Here's how the part is built. I have some questions about the finished solid (model axes, mm). A direction names the side the tool comes from. Round coordinates to 2 decimals unless told otherwise and drop trailing zeros. Order: outer loops, then holes, each group sorted by start corner. A loop starts at its lowest first (then second) coordinate and runs counter-clockwise, first axis right, second up.
```python
from build123d import *

# Parameters (mm, degrees)
BOSS_EXTRU_1_DEPTH      = 12
BOSS_EXTRU_1_DEPTH_BACK = 6
ENL_V_MAT_EXTRU_1_DEPTH = 168.845911478
BOSS_EXTRU_2_DEPTH      = 20
ENL_V_MAT_EXTRU_2_DEPTH = 169.042623851
ESQUISSE5_R             = 1.9
ENL_V_MAT_EXTRU_3_DEPTH = 10
CONG_1_R                = 3
CONG_2_R                = 1.5


with BuildPart() as part:
    # Esquisse1 → Boss.-Extru.1 (new, two sides: drawn at the far end of the back side and taken through both)
    with BuildSketch(Plane(origin=(0, 0, 0), x_dir=(1, 0, 0), z_dir=(0, 1, 0)).offset(-BOSS_EXTRU_1_DEPTH_BACK)):
        with BuildLine():
            Line((142.5, -81), (152.865954352, -81))
            ThreePointArc((152.865954352, -81), (158.655064541, -68.975144042), (163.5, -56.539808984))
            Line((163.5, -56.539808984), (163.5, -45))
            Line((163.5, -45), (155.5, -45))
            ThreePointArc((155.5, -45), (152.933130519, -53.072663298), (149.947490809, -61))
            Line((149.947490809, -61), (142.5, -61))
            Line((142.5, -61), (142.5, -81))
        make_face()
    extrude(amount=BOSS_EXTRU_1_DEPTH + BOSS_EXTRU_1_DEPTH_BACK)

    # Esquisse2 → Enlèv. mat.-Extru.1 (cut, through all)
    with BuildSketch(Plane.XY.offset(81)):
        Polygon((142.5, -6), (142.5, 12), (143.758682615, 12), align=None)
    extrude(amount=-ENL_V_MAT_EXTRU_1_DEPTH, mode=Mode.SUBTRACT)

    # Esquisse3 → Boss.-Extru.2 (add)
    with BuildSketch(Plane.XY.offset(81)):
        Polygon((143.758682615, 12), (143.933073799, 14.493910126), (150.916022151, 14.005614809), (150.916022151, 12), align=None)
    extrude(amount=-BOSS_EXTRU_2_DEPTH)

    # Esquisse4 → Enlèv. mat.-Extru.2 (cut, through all)
    with BuildSketch(Plane.XY.offset(81)):
        Polygon((142.5, -6), (143.235509062, 4.518269623), (145.5, -6), align=None)
    extrude(amount=-ENL_V_MAT_EXTRU_2_DEPTH, mode=Mode.SUBTRACT)

    # Esquisse5 → Enlèv. mat.-Extru.3 (cut)
    with BuildSketch(Plane(origin=(1.708954599, 24.439189363, 0), x_dir=(0.9975640502598248, -0.06975647374411768, 0), z_dir=(0.06975647374411768, 0.9975640502598248, 0))):
        with Locations(Location((146.571416004, -66, 0), (0, 0, 180))):
            Circle(ESQUISSE5_R)
        with Locations((146.571416004, -76)):
            Circle(ESQUISSE5_R)
    extrude(amount=-ENL_V_MAT_EXTRU_3_DEPTH, mode=Mode.SUBTRACT)

    # Esquisse7 → Enlèvement de matière-Révolution1 (revolve, cut)
    with BuildSketch(Plane(origin=(0, 0, 0), x_dir=(1, 0, 0), z_dir=(0, 1, 0)), mode=Mode.PRIVATE) as enl_vement_de_mati_re_r_volution1_sk:
        Polygon((156.5, -52.9), (160, -52.9), (160, -52.55), (163.5, -52.55), (163.5, -51), (150.916022151, -51), (150.916022151, -53.884605954), align=None)
    revolve(enl_vement_de_mati_re_r_volution1_sk.sketch.rotate(Axis((150.916022151, 0, 51), (-1, 0, 0)), 180), axis=Axis((150.916022151, 0, 51), (-1, 0, 0)), mode=Mode.SUBTRACT)

    # Congé1
    # the kernel refuses this fillet: 3 mm, written as the material it adds along each edge
    with BuildSketch(Plane(origin=(150.916022151, 12, 81), x_dir=(0, 1, 0), z_dir=(0, 0, -1))) as cong_1_piece_1_section:
        with BuildLine():
            CenterArc((3, 2.830405994), CONG_1_R, 180, 70.642479406)
            Line((0, 2.830405994), (0, 0))
            Line((0, 0), (2.005614809, 0))
        make_face()
    cong_1_piece_1 = extrude(amount=20, mode=Mode.PRIVATE)
    cong_1_piece_1 = cong_1_piece_1 & Plane(origin=(0, 12, 0), x_dir=(0.8836182332495415, 0, 0.46820809248555173), z_dir=(0, -1, 0)) * Cylinder(173, 52, mode=Mode.PRIVATE)
    add(cong_1_piece_1)
    with BuildSketch(Plane(origin=(149.947490809, 12, 61), x_dir=(-1, 0, 0), z_dir=(0, -1, 0))) as cong_1_piece_2:
        with BuildLine():
            CenterArc((2.032083033, 3), CONG_1_R, 201.410940908, 68.589059092)
            ThreePointArc((-0.760875339, 1.904836298), (-0.383454711, 0.95121301), (0, 0))
            Line((0, 0), (2.032083033, 0))
        make_face()
    extrude(amount=18)
    # the kernel refuses this fillet: 3 mm, written as the material it takes off along each edge
    with BuildSketch(Plane(origin=(163.5, 12, 69.289808984), x_dir=(0, -1, 0), z_dir=(0, 0, -1))) as cong_1_2_piece_1:
        with BuildLine():
            CenterArc((CONG_1_R, CONG_1_R), CONG_1_R, 180, 90)
            Line((0, CONG_1_R), (0, 0))
            Line((0, 0), (CONG_1_R, 0))
        make_face()
    extrude(amount=31.789808984, mode=Mode.SUBTRACT)
    with BuildSketch(Plane(origin=(155.5, 17.5970247, 45), x_dir=(-0.2845583113069487, 0, 0.9586587335783978), z_dir=(0, -1, 0))) as cong_1_2_piece_2:
        with BuildLine():
            CenterArc((2.238904242, -2.999929578), CONG_1_R, 90.392583202, 73.074968252)
            Line((-0.637071959, -2.146254644), (0, 0))
            ThreePointArc((0, 0), (1.109174397, -0.003799974), (2.218348794, 0))
        make_face()
    extrude(amount=29.194049399, mode=Mode.SUBTRACT)

    # Esquisse8 → Enlèvement de matière-Révolution2 (revolve, cut)
    with BuildSketch(Plane(origin=(0, 0, 0), x_dir=(1, 0, 0), z_dir=(0, 1, 0)), mode=Mode.PRIVATE) as enl_vement_de_mati_re_r_volution2_sk:
        Polygon((143.15277955, -61.193532862), (159.075453795, -68), (159.68470235, -66.574757495), (156.466412822, -65.199034952), (156.603985076, -64.877205999), (153.385695549, -63.501483455), (144.614610154, -57.773806881), align=None)
    revolve(enl_vement_de_mati_re_r_volution2_sk.sketch.rotate(Axis((0, 0, 0), (0.9195112936111692, 0, 0.3930635838150288)), 180), axis=Axis((0, 0, 0), (0.9195112936111692, 0, 0.3930635838150288)), mode=Mode.SUBTRACT)

    # Congé2
    cong_2_edges = [part.edges().sort_by_distance(p)[0] for p in [
        (145.330393567, 4.371781028, 76),
        (149.121136958, 4.106706428, 66),
        (143.325850505, 4.098645221, 61),
        (144.367754531, -0.740865188, 81),
        (145.212814743, -4.66606136, 61),
        (152.865954352, 3, 81),
    ]]
    fillet(cong_2_edges, radius=CONG_2_R)


solid = part.part
```
1) If we section it at B-B (y = 0.75): Give the number of separate pieces and of enclosed holes in the cut face, plus the area to 3 significant figures.
2) I'm going to push flat-ended pins straight in: pin 1 (8 mm diameter, centred on y = 6, z = 75.5, fed in from -X); pin 2 (5 mm diameter, centred on x = 153, y = 4.5, fed in from -Z); pin 3 (6 mm diameter, centred on y = 4.5, z = 72.5, fed in from +X); pin 4 (6 mm diameter, centred on x = 152.5, z = 71.5, fed in from +Y). Where does each tip first touch, or does it pass through?
3) If we section it at A-A (z = 51): Write out the boundary of the cut face in (x, y), plus the area to 3 significant figures.
4) I need wall thicknesses on line 1 (Y direction, x = 157.85, z = 51); line 2 (Z direction, x = 146.5, y = 7.25); line 3 (Z direction, x = 145.25, y = 8.5). Which ranges of each line are inside material? Lowest first, please.
5) For faces 5 (the flat face through (147, -4, 61)), 6 (the cylindrical face through (147.22, 10.063, 77.855)), which set-ups out of +Z, -Z, +X, -X, +Y, -Y let a thin tool reach every point of the face, with its end or its side?
6) We'd pull the mould along Y, two halves only. Please class faces 1 (the cylindrical face through (144.68, -0.15, 80.55)), 2 (the flat face through (149, 4, 81)), 3 (the cylindrical face through (158.274, -0.571, 49.188)), 4 (the cylindrical face through (161.774, 0.594, 49.568)): +Y half, -Y half, draft (parallel to the pull), parting line (faces both ways), or undercut.
7) If we section it at C-C (z = 72): Write out the boundary of the cut face in (x, y).
Solutions:
1. separate pieces: 3
1. enclosed holes: 0
1. area: 342 mm2
2. pin 1: stops at x = 143.24
2. pin 2: stops at z = 46
2. pin 3: stops at x = 158.43
2. pin 4: stops at y = 14.1
3. outline: (153.64, -6) - (163.5, -6) - (163.5, -1.55) - (160, -1.55) - (160, -1.9) - (156.5, -1.9) - (153.64, -2.4) - close; (153.64, 2.4) - (156.5, 1.9) - (160, 1.9) - (160, 1.55) - (163.5, 1.55) - (163.5, 9) arc R3 ccw to (160.5, 12) - (153.64, 12) - close
3. area: 139 mm2
4. line 1: y = -6 to -1.9, 1.9 to 12
4. line 2: z = 61 to 64.35, 67.65 to 74.35, 77.65 to 81
4. line 3: z = 61 to 81
5. face 5: -Z, -X, +Y, -Y
5. face 6: none
6. face 1: -Y half
6. face 2: draft
6. face 3: undercut
6. face 4: undercut
7. outline: (143.24, 4.52) - (145.5, -6) - (157.31, -6) - (157.31, 12) - (153.75, 12) arc R3 cw to (150.92, 14.01) - (143.93, 14.49) - close
